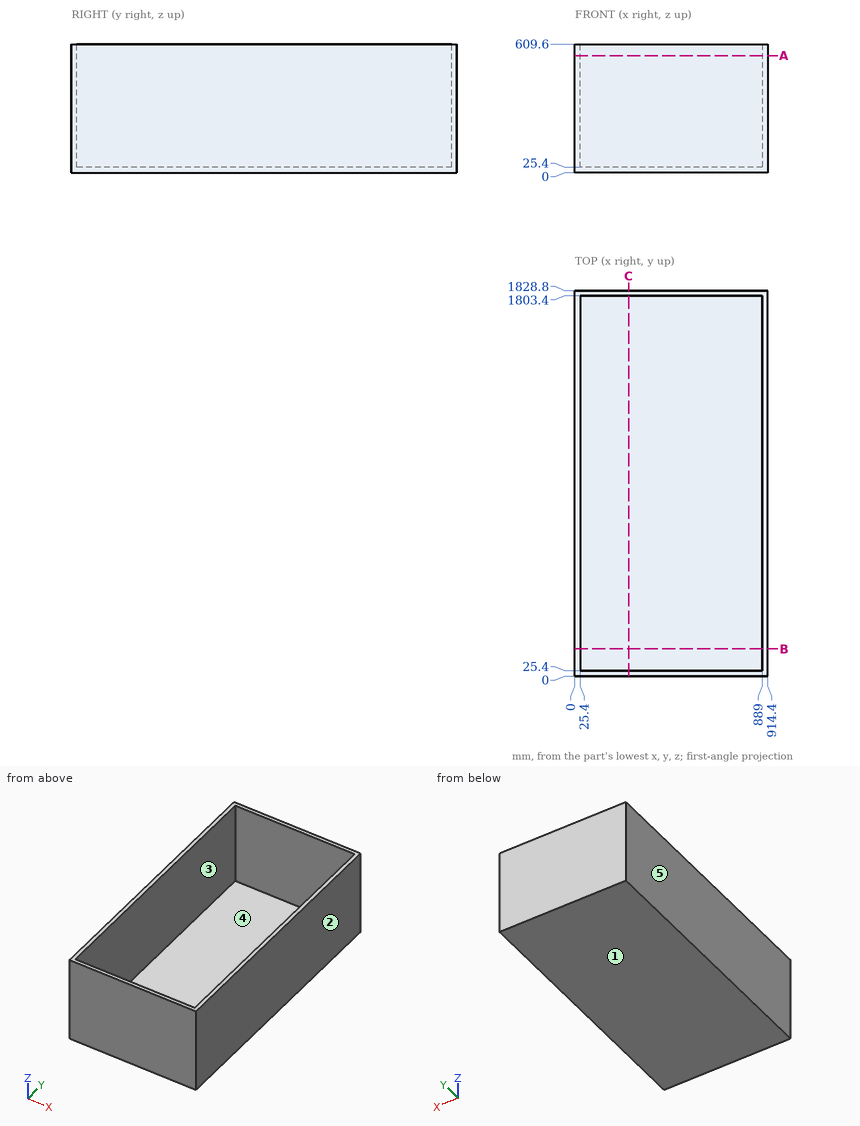
Geometry check sheet. Reference: drawing and pictorial views, mm from the part's lowest x, y, z. A direction names the side the tool comes from. Coordinates: 2 decimals unless noted, no trailing zeros. Write each loop counter-clockwise with the first axis right and the second up, starting at its lowest first coordinate (ties: lowest second). Pieces come first, ordered by that corner, then holes. Notation, with made-up numbers: (49.5, 87.25) - (91.5, 87.25) arc R20 cw to (91.5, 116.25) - close; hole circle Ø11 at (40.5, 7.25). An arc over 180 degrees is marked (long way). Write item = value, one per line.
Q1. Go/stop test with a flat-tipped pin: pin 1 Ø10 at (x, y) = (272, 901) entering from +Z. Record where the tip stops, or that it passes through.
Answer:
pin_1 = 25.4
Q2. Mould release check, pull along X, two halves, no side actions. Record for the marked faces 1, 2 and 3: released by +X, released by -X, zero draft, split by the parting line, or undercut.
Answer:
face_1 = zero draft
face_2 = released by +X
face_3 = undercut
Q3. Access from +Z, -Z, +X, -X, +Y, -Y to the whole of each face (thin tool, end or side, straight path). Record for the marked faces 4 and 5.
Answer:
face_4 = +Z
face_5 = +Z, -Z, -X, +Y, -Y
Q4. Cross-section at A-A (z = 555). Enter the section's corners in (x, y), plus the area to 3 significant figures.
Answer:
outline = (0, 0) - (914.4, 0) - (914.4, 1828.8) - (0, 1828.8) - close; hole (25.4, 25.4) - (889, 25.4) - (889, 1803.4) - (25.4, 1803.4) - close
area = 137,000 mm²
Q5. Cross-section at C-C (x = 255.5). Enter the section's corners in (y, z), plus the area to 3 significant figures.
Answer:
outline = (0, 0) - (1828.8, 0) - (1828.8, 609.6) - (1803.4, 609.6) - (1803.4, 25.4) - (25.4, 25.4) - (25.4, 609.6) - (0, 609.6) - close
area = 76,100 mm²
Q6. Material ranges on L1, parallel to X at y = 83, z = 46.5; L2, parallel to Y at x = 208.5, z = 470; L3, parallel to Z at x = 231, y = 207.5, recorded low to high. Write a range as from..to.
Answer:
L1 = 0..25.4, 889..914.4
L2 = 0..25.4, 1803.4..1828.8
L3 = 0..25.4
Q7. Cross-section at B-B (y = 129). Enter the section's corners in (x, z), plus the area to 3 significant figures.
Answer:
outline = (0, 0) - (914.4, 0) - (914.4, 609.6) - (889, 609.6) - (889, 25.4) - (25.4, 25.4) - (25.4, 609.6) - (0, 609.6) - close
area = 52,900 mm²
